Design review of the part built by this model. Coordinates are the model's own, in mm. A direction names the side the tool comes from. Coordinates: 2 decimals unless noted, no trailing zeros. Loops run counter-clockwise (first coordinate to the right, second up) from the corner with the lowest first, then second, coordinate; pieces in that order, holes last.
from build123d import *

# Parameters (mm, degrees)
BOSS_EXTRUDE1_START = -17
BOSS_EXTRUDE1_DEPTH = 35
SKETCH2_R           = 10.45
CUT_EXTRUDE1_DEPTH  = 32
SKETCH3_R           = 6.5
CUT_EXTRUDE2_DEPTH  = 62.814237842
SKETCH4_R           = 12.5
CUT_EXTRUDE3_DEPTH  = 64.419239983
FILLET5_R           = 10
FILLET6_R           = 10


with BuildPart() as part:
    # Sketch1 → Boss-Extrude1 (new body)
    with BuildSketch(Plane.YZ.offset(BOSS_EXTRUDE1_START)):
        with BuildLine():
            Line((-14, 0), (-14, 51))
            Line((-14, 51), (14, 51))
            Line((14, 51), (14, 0))
            ThreePointArc((14, 0), (0, -14), (-14, 0))
        make_face()
    extrude(amount=BOSS_EXTRUDE1_DEPTH)

    # Sketch2 → Cut-Extrude1 (cut)
    with BuildSketch(Plane.YZ.offset(18)):
        with Locations(Location((0, 0, 0), (0, 0, 270))):
            Circle(SKETCH2_R)
    extrude(amount=-CUT_EXTRUDE1_DEPTH, mode=Mode.SUBTRACT)

    # Sketch3 → Cut-Extrude2 (cut, through all)
    with BuildSketch(Plane.YZ.offset(-14)):
        with Locations(Location((0, 0, 0), (0, 0, 270))):
            Circle(SKETCH3_R)
    extrude(amount=-CUT_EXTRUDE2_DEPTH, mode=Mode.SUBTRACT)

    # Sketch4 → Cut-Extrude3 (cut, through all)
    with BuildSketch(Plane.YZ.offset(18)):
        with Locations(Location((0, 35.95, 0), (0, 0, 270))):
            Circle(SKETCH4_R)
    extrude(amount=-CUT_EXTRUDE3_DEPTH, mode=Mode.SUBTRACT)

    # Fillet5
    fillet5_edges = [part.edges().sort_by_distance(p)[0] for p in [
        (0.5, 14, 51),
    ]]
    fillet(fillet5_edges, radius=FILLET5_R)

    # Fillet6
    fillet6_edges = [part.edges().sort_by_distance(p)[0] for p in [
        (0.5, -14, 51),
    ]]
    fillet(fillet6_edges, radius=FILLET6_R)


solid = part.part
Q1. Take a section at A-A, the plane y = 0. Write out the cut boundary in (x, z).
Q2. Take a section at D-D, the plane y = -9.5. Write out the cut boundary in (x, z), then the cut area to 3 significant figures.
Q3. For line 1 (Y direction, x = -16, z = 0); line 2 (Z direction, x = -3, y = -8.75); line 3 (Y direction, x = 8, z = 35.95), list the stretches that pass through material, from the lowest coordinate up.
Q4. Take a section at C-C, the plane x = -13. Write out the cut boundary in (y, z), then the cut area to 3 significant figures.
Q5. Clearance check with flat-ended pins moving along their axes: pin 1 Ø15 at (y, z) = (0, 0) entering from -X; pin 2 Ø6 at (x, y) = (5, 9.5) entering from +Z; pin 3 Ø4 at (x, y) = (-12.5, 6.5) entering from -Z; pin 4 Ø5 at (x, y) = (2.5, 9) entering from -Z. State where each tip first meets the part, or that it passes through.
Q6. Machinability: for faces 5 (the cylindrical face through (0.75, 10.99, 48.15)), 6 (the cylindrical face through (2.224, 3.139, -9.967)), which of the approach directions +Z, -Z, +X, -X, +Y, -Y give a long, thin tool a straight path to every point of the face, cutting with its end or side? Answer none if there is none.
Q7. Take a section at B-B, the plane z = 35.95. Write out the cut boundary in (x, y), then the cut area to 3 significant figures.
Q8. The part is to be moulded in two halves that separate along Y. For faces 1 (the flat face through (-14, 0, -7)), 2 (the flat face through (-17, 0, 12)), 3 (the flat face through (0, 14, 21)), 4 (the flat face through (0, -14, 20)), say which applies: pulls with the +Y half, pulls with the -Y half, needs draft (parallel to the pull), parting line crosses it, or undercut.
Entries:
1. outline: (-17, -14) - (18, -14) - (18, -10.45) - (-14, -10.45) - (-14, -6.5) - (-17, -6.5) - close; (-17, 6.5) - (-14, 6.5) - (-14, 10.45) - (18, 10.45) - (18, 23.45) - (-17, 23.45) - close; (-17, 48.45) - (18, 48.45) - (18, 51) - (-17, 51) - close
2. outline: (-17, -10.28) - (18, -10.28) - (18, -4.35) - (-14, -4.35) - (-14, 4.35) - (18, 4.35) - (18, 27.83) - (-17, 27.83) - close; (-17, 44.07) - (18, 44.07) - (18, 49.35) - (-17, 49.35) - close
2. area: 1,240 mm2
3. line 1: y = -14 to -6.5, 6.5 to 14
3. line 2: z = -10.93 to -5.71, 5.71 to 27.02, 44.88 to 49.8
3. line 3: y = -14 to -12.5, 12.5 to 14
4. outline: (-14, 0) arc R14 ccw to (14, 0) - (14, 41) arc R10 ccw to (4, 51) - (-4, 51) arc R10 ccw to (-14, 41) - close; hole circle Ø25 at (0, 35.95); hole circle Ø20.9 at (0, 0)
4. area: 859 mm2
5. pin 1: stops at x = -17
5. pin 2: stops at z = 50.68
5. pin 3: stops at z = -13.26
5. pin 4: stops at z = -12.4
6. face 5: +Z, +X, -X, +Y
6. face 6: +X
7. outline: (-17, -14) - (18, -14) - (18, -12.5) - (-17, -12.5) - close; (-17, 12.5) - (18, 12.5) - (18, 14) - (-17, 14) - close
7. area: 105 mm2
8. face 1: undercut
8. face 2: needs draft
8. face 3: pulls with the +Y half
8. face 4: pulls with the -Y half
